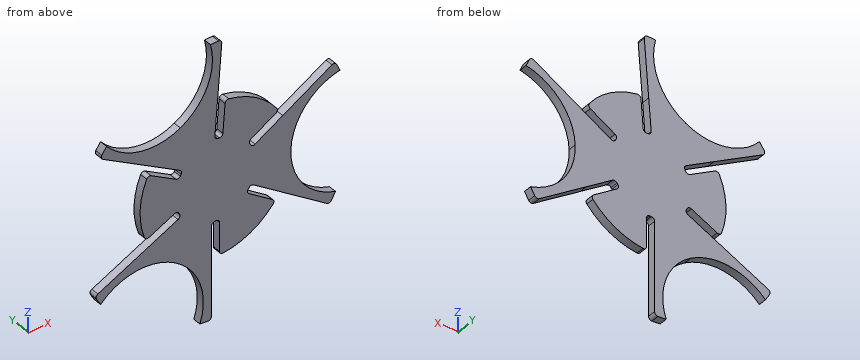
from build123d import *

# Parameters (mm, degrees)
EXTRUDE_1_DEPTH = 5
EXTRUDE_2_DEPTH = 5
FILLET_1_R      = 2


with BuildPart() as part:
    # 草圖1 → 填料-伸長1 (new body)
    with BuildSketch(Plane(origin=(0, 0, 0), x_dir=(1, 0, 0), z_dir=(0, 1, 0))):
        with BuildLine():
            Line((41.895571715, -21.301668261), (22.900635095, -10.334936491))
            Line((22.900635095, -10.334936491), (20.400635095, -14.665063509))
            Line((20.400635095, -14.665063509), (39.395571715, -25.63179528))
            ThreePointArc((39.395571715, -25.63179528), (25.066666667, -39.75754296), (6.143670641, -46.596730691))
            Line((6.143670641, -46.596730691), (4.437329437, -24.729741355))
            Line((4.437329437, -24.729741355), (-0.547516958, -25.118722602))
            Line((-0.547516958, -25.118722602), (1.158824246, -46.985711938))
            ThreePointArc((1.158824246, -46.985711938), (-21.897708862, -41.587141602), (-39.395571715, -25.63179528))
            Line((-39.395571715, -25.63179528), (-20.400635095, -14.665063509))
            Line((-20.400635095, -14.665063509), (-22.900635095, -10.334936491))
            Line((-22.900635095, -10.334936491), (-41.895571715, -21.301668261))
            ThreePointArc((-41.895571715, -21.301668261), (-46.964375529, -1.829598641), (-43.425787832, 17.977790497))
            Line((-43.425787832, 17.977790497), (-23.635248961, 8.522030659))
            Line((-23.635248961, 8.522030659), (-21.479693405, 13.033524896))
            Line((-21.479693405, 13.033524896), (-41.270232276, 22.489284734))
            ThreePointArc((-41.270232276, 22.489284734), (-25.066666667, 39.75754296), (-2.5, 46.933463541))
            Line((-2.5, 46.933463541), (-2.5, 25))
            Line((-2.5, 25), (2.5, 25))
            Line((2.5, 25), (2.5, 46.933463541))
            ThreePointArc((2.5, 46.933463541), (21.897708862, 41.587141602), (37.282117191, 28.618940193))
            Line((37.282117191, 28.618940193), (19.197919523, 16.207710695))
            Line((19.197919523, 16.207710695), (22.027210363, 12.085197706))
            Line((22.027210363, 12.085197706), (40.111408031, 24.496427205))
            ThreePointArc((40.111408031, 24.496427205), (46.964375529, 1.829598641), (41.895571715, -21.301668261))
        make_face()
    extrude(amount=-EXTRUDE_1_DEPTH)

    # 草圖2 → 填料-伸長2 (add)
    with BuildSketch(Plane(origin=(0, 0, 0), x_dir=(1, 0, 0), z_dir=(0, 1, 0))):
        with BuildLine():
            ThreePointArc((-21.897708534, -41.587141774), (-31.667962065, -34.729528915), (-39.395571715, -25.63179528))
            Line((-39.395571715, -25.63179528), (-71.897112041, -44.396568337))
            ThreePointArc((-71.897112041, -44.396568337), (-69.935607979, -47.426371742), (-67.846508155, -50.369646923))
            ThreePointArc((-67.846508155, -50.369646923), (-46.409467113, -37.935155113), (-21.897708534, -41.587141774))
        make_face()
        with BuildLine():
            ThreePointArc((1.158824246, -46.985711938), (-10.715011448, -45.76230468), (-21.897708534, -41.587141774))
            ThreePointArc((-21.897708534, -41.587141774), (-5.016457748, -59.73064391), (-3.138403923, -84.441698353))
            ThreePointArc((-3.138403923, -84.441698353), (0.470468308, -84.498690283), (4.078482182, -84.401516474))
            Line((4.078482182, -84.401516474), (1.158824246, -46.985711938))
        make_face()
        with BuildLine():
            ThreePointArc((46.964375577, 1.829597397), (45.910635161, -10.060495966), (41.895571715, -21.301668261))
            Line((41.895571715, -21.301668261), (74.397112041, -40.066441318))
            ThreePointArc((74.397112041, -40.066441318), (76.040246727, -36.852827268), (77.544647892, -33.571976159))
            ThreePointArc((77.544647892, -33.571976159), (56.057542109, -21.224200551), (46.964375577, 1.829597397))
        make_face()
        with BuildLine():
            ThreePointArc((40.111408031, 24.496427205), (44.988824347, 13.601679451), (46.964375577, 1.829597397))
            ThreePointArc((46.964375577, 1.829597397), (54.236483405, 25.520941458), (74.697857874, 39.502911652))
            ThreePointArc((74.697857874, 39.502911652), (72.942778218, 42.656782648), (71.054616293, 45.732827415))
            Line((71.054616293, 45.732827415), (40.111408031, 24.496427205))
        make_face()
        with BuildLine():
            ThreePointArc((-25.066667605, 39.757542368), (-14.242673622, 44.79002398), (-2.5, 46.933463541))
            Line((-2.5, 46.933463541), (-2.5, 84.463009655))
            ThreePointArc((-2.5, 84.463009655), (-6.104638749, 84.27919901), (-9.698139737, 83.941623082))
            ThreePointArc((-9.698139737, 83.941623082), (-9.648074589, 59.159354704), (-25.066667605, 39.757542368))
        make_face()
        with BuildLine():
            ThreePointArc((-41.270232276, 22.489284734), (-34.273812918, 32.160624187), (-25.066667605, 39.757542368))
            ThreePointArc((-25.066667605, 39.757542368), (-49.220026504, 34.209701843), (-71.559453951, 44.938786701))
            ThreePointArc((-71.559453951, 44.938786701), (-73.413246526, 41.841907635), (-75.133098475, 38.668689059))
            Line((-75.133098475, 38.668689059), (-41.270232276, 22.489284734))
        make_face()
    extrude(amount=-EXTRUDE_2_DEPTH)

    # 圓角1
    fillet_1_edges = [part.edges().sort_by_distance(p)[0] for p in [
        (71.054616293, -2.5, -45.732827415),
        (-2.5, -2.5, -84.463009655),
        (-75.133098475, -2.5, -38.668689059),
        (4.437329437, -2.5, 24.729741355),
        (-0.547516958, -2.5, 25.118722602),
        (-20.400635095, -2.5, 14.665063509),
        (-22.900635095, -2.5, 10.334936491),
        (-41.895571715, -2.5, 21.301668261),
        (-43.425787832, -2.5, -17.977790497),
        (-23.635248961, -2.5, -8.522030659),
        (-21.479693405, -2.5, -13.033524896),
        (-2.5, -2.5, -25),
        (2.5, -2.5, -25),
        (2.5, -2.5, -46.933463541),
        (37.282117191, -2.5, -28.618940193),
        (19.197919523, -2.5, -16.207710695),
        (22.027210363, -2.5, -12.085197706),
        (22.900635095, -2.5, 10.334936491),
        (20.400635095, -2.5, 14.665063509),
        (39.395571715, -2.5, 25.63179528),
        (6.143670641, -2.5, 46.596730691),
        (-71.897112041, -2.5, 44.396568337),
        (4.078482182, -2.5, 84.401516474),
        (74.397112041, -2.5, 40.066441318),
    ]]
    fillet(fillet_1_edges, radius=FILLET_1_R)


solid = part.part
CAD build for the part. Positions are in the model's coordinates, mm. Give positions to 0.01 mm unless a question says otherwise; leave off trailing zeros. Order: outer loops, then holes, each group sorted by start corner. A loop starts at its lowest first (then second) coordinate and runs counter-clockwise, first axis right, second up. Notation, with made-up numbers: (70.5, 81) -> (108.5, 81) arc R20 cw to (108.5, 100) -> close; hole circle Ø1 at (-22, -7.75). An arc over 180 degrees is marked (long way). Return JSON: item names as keys, results as strings.
Q1. Saw through at B-B (x = -49). Write the cut outline in (y, z).
Working result:
{"outline": "(-5, -34.19) -> (0, -34.19) -> (0, -26.18) -> (-5, -26.18) -> close; (-5, 31.18) -> (0, 31.18) -> (0, 38.53) -> (-5, 38.53) -> close"}
Q2. Saw through at A-A (x = 33.5). Write the cut outline in (y, z), then the cut area to 3 significant figures.
Working result:
{"outline": "(-5, -32.97) -> (0, -32.97) -> (0, -26.02) -> (-5, -26.02) -> close; (-5, -19.96) -> (0, -19.96) -> (0, 16.45) -> (-5, 16.45) -> close; (-5, 22.23) -> (0, 22.23) -> (0, 32.97) -> (-5, 32.97) -> close", "area": "270 mm²"}
Q3. Saw through at D-D (z = -56.5). Write the cut outline in (x, y).
Working result:
{"outline": "(-10.69, -5) -> (-2.5, -5) -> (-2.5, 0) -> (-10.69, 0) -> close"}
Q4. Drill centre lines: line 1 (Z direction, x = 32, y = -0.9); line 2 (X direction, y = -2.4, z = -32); line 3 (X direction, y = -2.4, z = 19). Where is each one in solid material? Low to high.
Working result:
{"line 1": "-34.42 to -24.99, -18.93 to 15.59, 21.36 to 34.42", "line 2": "-61.18 to -2.5, 2.5 to 34.42, 51.04 to 60.31", "line 3": "-42.99 to -37.91, -27.91 to 27.91, 37.91 to 54.28"}
Q5. Flat gauge pins, fed straight in: pin 1 (1 mm diameter, centred on y = -2, z = -31, fed in from -X); pin 2 (2 mm diameter, centred on x = -10.5, y = -3, fed in from +Z); pin 3 (3 mm diameter, centred on y = -2, z = -61, fed in from -X). Where does each tip first touch, or does it go through?
Working result:
{"pin 1": "x = -60.13", "pin 2": "z = 52.1", "pin 3": "x = -9.53"}
Q6. Saw through at C-C (z = 59.5). Write the cut outline in (x, y).
Working result:
{"outline": "(-5.12, -5) -> (2.14, -5) -> (2.14, 0) -> (-5.12, 0) -> close"}
